For this review, take the finished solid that the model builds, in its own axes (mm). A direction names the side the tool comes from. Coordinates: 2 decimals unless noted, no trailing zeros. Order: outer loops, then holes, each group sorted by start corner. A loop starts at its lowest first (then second) coordinate and runs counter-clockwise, first axis right, second up. Notation, with made-up numbers: (53.25, 79.25) -> (64.25, 79.25) arc R25 cw to (64.25, 95.25) -> close; hole circle Ø1 at (27, 5.5). An arc over 180 degrees is marked (long way). Answer as a JSON object with one key per item and string values. Group by question number.
1) Add section B-B, the plane x = 11. Write out the cut boundary in (y, z).
2) For pin 1 (3 mm diameter, centred on x = 29.5, z = 77, fed in from -Y); pin 2 (0.9 mm diameter, centred on y = 9, z = 79.5, fed in from +X); pin 3 (1.2 mm diameter, centred on y = 12.5, z = 77, fed in from +X); pin 4 (4 mm diameter, centred on x = -2, y = 20, fed in from -Z), all flat-tipped, find the tip position at first contact; note any pin that passes through.
3) Add section A-A, the plane z = 77.25. Write out the cut boundary in (x, y).
4) Add section C-C, the plane y = 13.75. Write out the cut boundary in (x, z).
5) Wall thickness on L1, parallel to Y at x = -22.5, z = 79.05; L2, parallel to X at y = 12.5, z = 75.6; L3, parallel to Z at x = 15, y = 25.75: over which ranges is each line inside the solid? List them lowest first.
6) Draft analysis for pull direction Y (two halves, no side actions). For faces 4 (the conical face through (-19.607, 25.776, 79.635)), 5 (the conical face through (-34.542, 33.199, 79.865)), 6 (the flat face through (0, 16, 80)), 7 (the conical face through (-28.593, 18.724, 79.635)), state which applies: +Y half, -Y half, draft (parallel to the pull), parting line (faces both ways), or undercut.
7) Machinability: for faces 1 (the cylindrical face through (34.859, 33.397, 78.942)), 2 (the cylindrical face through (28.5, 18.82, 78.94)), 3 (the conical face through (19.574, 25.743, 79.635)), which of the approach directions +Z, -Z, +X, -X, +Y, -Y give a long, thin tool a straight path to every point of the face, cutting with its end or side? Answer none if there is none.
from build123d import *

# Parameters (mm, degrees)
BOSS_EXTRUDE1_START = 78.4
BOSS_EXTRUDE1_DEPTH = 1.6
CHAMFER1_SIZE       = 0.5
BOSS_EXTRUDE2_START = 78
BOSS_EXTRUDE2_DEPTH = 3
CHAMFER2_SIZE       = 0.5
BOSS_EXTRUDE3_START = 78
BOSS_EXTRUDE3_DEPTH = 3
CHAMFER3_SIZE       = 0.5
BOSS_EXTRUDE4_START = 78
BOSS_EXTRUDE4_DEPTH = 3
CHAMFER4_SIZE       = 0.5
BOSS_EXTRUDE5_START = 79.2
SKETCH5_W           = 3
SKETCH5_H           = 0.9
BOSS_EXTRUDE5_DEPTH = 0.9
BOSS_EXTRUDE6_START = -32
BOSS_EXTRUDE6_DEPTH = 4
BOSS_EXTRUDE7_START = 28
BOSS_EXTRUDE7_DEPTH = 4


with BuildPart() as part:
    # Sketch1 → Boss-Extrude1 (new body)
    with BuildSketch(Plane.XY.offset(BOSS_EXTRUDE1_START)):
        with BuildLine():
            Line((-32, 8.6), (32, 8.6))
            ThreePointArc((32, 8.6), (34.828427125, 9.771572875), (36, 12.6))
            Line((36, 12.6), (36, 30.6))
            ThreePointArc((36, 30.6), (34.828427125, 33.428427125), (32, 34.6))
            Line((32, 34.6), (-32, 34.6))
            ThreePointArc((-32, 34.6), (-34.828427125, 33.428427125), (-36, 30.6))
            Line((-36, 30.6), (-36, 12.6))
            ThreePointArc((-36, 12.6), (-34.828427125, 9.771572875), (-32, 8.6))
        make_face()
    extrude(amount=BOSS_EXTRUDE1_DEPTH)

    # Chamfer1
    chamfer1_edges = [part.edges().sort_by_distance(p)[0] for p in [
        (34.828427125, 9.771572875, 80),
        (36, 21.6, 80),
        (34.828427125, 33.428427125, 80),
        (0, 34.6, 80),
        (-34.828427125, 33.428427125, 80),
        (-36, 21.6, 80),
        (-34.828427125, 9.771572875, 80),
        (0, 8.6, 80),
    ]]
    chamfer(chamfer1_edges, length=CHAMFER1_SIZE)


with BuildPart() as body_2:
    # Sketch2 → Boss-Extrude2 (new body)
    with BuildSketch(Plane.XY.offset(BOSS_EXTRUDE2_START)):
        with BuildLine():
            Line((-3, 18.25), (3, 18.25))
            ThreePointArc((3, 18.25), (4.414213562, 18.835786438), (5, 20.25))
            Line((5, 20.25), (5, 24.25))
            ThreePointArc((5, 24.25), (4.414213562, 25.664213562), (3, 26.25))
            Line((3, 26.25), (-3, 26.25))
            ThreePointArc((-3, 26.25), (-4.414213562, 25.664213562), (-5, 24.25))
            Line((-5, 24.25), (-5, 20.25))
            ThreePointArc((-5, 20.25), (-4.414213562, 18.835786438), (-3, 18.25))
        make_face()
    extrude(amount=BOSS_EXTRUDE2_DEPTH)


with BuildPart() as part_1:
    add(part.part)

    # Combine1: cut body 2
    add(body_2.part, mode=Mode.SUBTRACT)

    # Chamfer2
    chamfer2_edges = [part_1.edges().sort_by_distance(p)[0] for p in [
        (-4.414213562, 18.835786438, 80),
        (0, 18.25, 80),
        (4.414213562, 18.835786438, 80),
        (5, 22.25, 80),
        (4.414213562, 25.664213562, 80),
        (0, 26.25, 80),
        (-4.414213562, 25.664213562, 80),
        (-5, 22.25, 80),
    ]]
    chamfer(chamfer2_edges, length=CHAMFER2_SIZE)


with BuildPart() as body_2_2:
    # Sketch3 → Boss-Extrude3 (new body)
    with BuildSketch(Plane.XY.offset(BOSS_EXTRUDE3_START)):
        with BuildLine():
            Line((21.1, 18.25), (27.1, 18.25))
            ThreePointArc((27.1, 18.25), (28.514213562, 18.835786438), (29.1, 20.25))
            Line((29.1, 20.25), (29.1, 24.25))
            ThreePointArc((29.1, 24.25), (28.514213562, 25.664213562), (27.1, 26.25))
            Line((27.1, 26.25), (21.1, 26.25))
            ThreePointArc((21.1, 26.25), (19.685786438, 25.664213562), (19.1, 24.25))
            Line((19.1, 24.25), (19.1, 20.25))
            ThreePointArc((19.1, 20.25), (19.685786438, 18.835786438), (21.1, 18.25))
        make_face()
    extrude(amount=BOSS_EXTRUDE3_DEPTH)


with BuildPart() as part_2:
    add(part_1.part)

    # Combine2: cut body 2 2
    add(body_2_2.part, mode=Mode.SUBTRACT)

    # Chamfer3
    chamfer3_edges = [part_2.edges().sort_by_distance(p)[0] for p in [
        (19.685786438, 18.835786438, 80),
        (24.1, 18.25, 80),
        (28.514213562, 18.835786438, 80),
        (29.1, 22.25, 80),
        (28.514213562, 25.664213562, 80),
        (24.1, 26.25, 80),
        (19.685786438, 25.664213562, 80),
        (19.1, 22.25, 80),
    ]]
    chamfer(chamfer3_edges, length=CHAMFER3_SIZE)


with BuildPart() as body_2_3:
    # Sketch4 → Boss-Extrude4 (new body)
    with BuildSketch(Plane.XY.offset(BOSS_EXTRUDE4_START)):
        with BuildLine():
            Line((-27.1, 18.25), (-21.1, 18.25))
            ThreePointArc((-21.1, 18.25), (-19.685786438, 18.835786438), (-19.1, 20.25))
            Line((-19.1, 20.25), (-19.1, 24.25))
            ThreePointArc((-19.1, 24.25), (-19.685786438, 25.664213562), (-21.1, 26.25))
            Line((-21.1, 26.25), (-27.1, 26.25))
            ThreePointArc((-27.1, 26.25), (-28.514213562, 25.664213562), (-29.1, 24.25))
            Line((-29.1, 24.25), (-29.1, 20.25))
            ThreePointArc((-29.1, 20.25), (-28.514213562, 18.835786438), (-27.1, 18.25))
        make_face()
    extrude(amount=BOSS_EXTRUDE4_DEPTH)


with BuildPart() as part_3:
    add(part_2.part)

    # Combine3: cut body 2 3
    add(body_2_3.part, mode=Mode.SUBTRACT)

    # Chamfer4
    chamfer4_edges = [part_3.edges().sort_by_distance(p)[0] for p in [
        (-28.514213562, 18.835786438, 80),
        (-24.1, 18.25, 80),
        (-19.685786438, 18.835786438, 80),
        (-19.1, 22.25, 80),
        (-19.685786438, 25.664213562, 80),
        (-24.1, 26.25, 80),
        (-28.514213562, 25.664213562, 80),
        (-29.1, 22.25, 80),
    ]]
    chamfer(chamfer4_edges, length=CHAMFER4_SIZE)


with BuildPart() as body_2_4:
    # Sketch5 → Boss-Extrude5 (new body)
    with BuildSketch(Plane.XY.offset(BOSS_EXTRUDE5_START)):
        with Locations((0, 8.95)):
            Rectangle(SKETCH5_W, SKETCH5_H)
    extrude(amount=BOSS_EXTRUDE5_DEPTH)


with BuildPart() as part_4:
    add(part_3.part)

    # Combine4: cut body 2 4
    add(body_2_4.part, mode=Mode.SUBTRACT)

    # Sketch6 → Boss-Extrude6 (add)
    with BuildSketch(Plane(origin=(0, 0, 0), x_dir=(0, 0, -1), z_dir=(1, 0, 0)).offset(BOSS_EXTRUDE6_START)):
        Polygon((-78.41, 12), (-74.6, 12), (-74.6, 12.8), (-74.9, 13.1), (-75.2, 13.1), (-75.2, 12.8), (-78.41, 12.8), align=None)
    extrude(amount=BOSS_EXTRUDE6_DEPTH)

    # Sketch7 → Boss-Extrude7 (add)
    with BuildSketch(Plane(origin=(0, 0, 0), x_dir=(0, 0, -1), z_dir=(1, 0, 0)).offset(BOSS_EXTRUDE7_START)):
        Polygon((-78.41, 12), (-74.6, 12), (-74.6, 12.8), (-74.9, 13.1), (-75.2, 13.1), (-75.2, 12.8), (-78.41, 12.8), align=None)
    extrude(amount=BOSS_EXTRUDE7_DEPTH)


solid = part_4.part
Output values:
{
 "1": {"outline": "(8.6, 78.4) -> (34.6, 78.4) -> (34.6, 79.5) -> (34.1, 80) -> (9.1, 80) -> (8.6, 79.5) -> close"},
 "2": {"pin 1": "stops at y = 8.6", "pin 2": "stops at x = 34.47", "pin 3": "stops at x = 32", "pin 4": "stops at z = 78.4"},
 "3": {"outline": "(-32, 12) -> (-28, 12) -> (-28, 12.8) -> (-32, 12.8) -> close; (28, 12) -> (32, 12) -> (32, 12.8) -> (28, 12.8) -> close"},
 "4": {"outline": "(-36, 78.4) -> (36, 78.4) -> (36, 79.5) -> (35.5, 80) -> (-35.5, 80) -> (-36, 79.5) -> close"},
 "5": {"L1": "y = 8.6 to 18.25, 26.25 to 34.6", "L2": "x = -32 to -28, 28 to 32", "L3": "z = 78.4 to 80"},
 "6": {"face 4": "undercut", "face 5": "+Y half", "face 6": "draft", "face 7": "undercut"},
 "7": {"face 1": "+Z, -Z, +X, +Y", "face 2": "+Z, -Z", "face 3": "+Z"}
}
